```python
from build123d import *

# Parameters (mm, degrees)
F1_DEPTH = 10
F2_W     = 10
F2_H     = 10
F3_DEPTH = 5


with BuildPart() as f1:
    # F0 (on Right) → F1 (new body)
    with BuildSketch(Plane.YZ):
        Polygon((0, -4.91692), (0, 0), (-500, 0), (0, -500), (0, -492.686017), (-487.769097, -4.91692), align=None)
    extrude(amount=F1_DEPTH)

    # F2 (on face) → F3 (join)
    with BuildSketch(Plane.XY):
        with Locations((5, -495)):
            Rectangle(F2_W, F2_H)
    extrude(amount=F3_DEPTH)


solid = f1.part
```
Source: CAD feature listing. Evaluate the final solid. Frame: model axes, mm. Coordinates: 2 decimals unless noted, no trailing zeros. Order: outer loops, then holes, each group sorted by start corner. A loop starts at its lowest first (then second) coordinate and runs counter-clockwise, first axis right, second up. Notation, with made-up numbers: (55.25, 49) - (84.25, 49) arc R24 cw to (84.25, 83) - close; hole circle Ø8 at (87, 54). An arc over 180 degrees is marked (long way). One line per item, written item: value.
1) Mould query, pull axis Z, two halves, no side actions, for faces 1 (the face through (4.93, -240.47, -252.216)), 2 (the face through (5, -253, -247)), 3 (the face through (10, -381, -118)). Classes: released by +Z, released by -Z, zero draft, split by the parting line, or undercut.
Computed values:
face 1: undercut
face 2: released by -Z
face 3: zero draft
2) Contact query for flat-ended pins moving along their axis: pin 1 (1.5 mm diameter, centred on x = 4.5, z = -392.5, fed in from -Y); pin 2 (1.5 mm diameter, centred on x = 4.5, z = -385.5, fed in from -Y); pin 3 (5 mm diameter, centred on x = 5, y = -270.5, fed in from -Z). Output: stop coordinate, or through.
Computed values:
pin 1: stops at y = -108.25
pin 2: stops at y = -115.25
pin 3: stops at z = -232
3) Cut plane A-A on y = -228. Output: boundary loops of the cut face in (x, z).
Computed values:
outline: (0, -272) - (10, -272) - (10, -264.69) - (0, -264.69) - close; (0, -4.92) - (10, -4.92) - (10, 0) - (0, 0) - close
4) Cut plane C-C on z = -295. Output: boundary loops of the cut face in (x, y).
Computed values:
outline: (0, -205) - (10, -205) - (10, -197.69) - (0, -197.69) - close
5) Cut plane B-B on x = 1.5. Output: boundary loops of the cut face in (y, z).
Computed values:
outline: (-500, 0) - (0, -500) - (0, -492.69) - (-487.77, -4.92) - (0, -4.92) - (0, 0) - (-490, 0) - (-490, 5) - (-500, 5) - close
6) Ray query, line 1 (Z direction, x = 0.75, y = -37.5); line 2 (Z direction, x = 4, y = -63); line 3 (Y direction, x = 1, z = -395.5). Return the intervals inside material, ascending. Write a range as [from, to].
Computed values:
line 1: z = [-462.5, -455.19], [-4.92, 0]
line 2: z = [-437, -429.69], [-4.92, 0]
line 3: y = [-104.5, -97.19]
